Source: CAD feature listing. Evaluate the final solid. Frame: model axes, mm. A direction names the side the tool comes from. Round coordinates to 2 decimals unless told otherwise and drop trailing zeros. Loops run counter-clockwise (first coordinate to the right, second up) from the corner with the lowest first, then second, coordinate; pieces in that order, holes last. Notation, with made-up numbers: (28, 41) -> (39, 41) arc R22 ccw to (39, 50) -> close; hole circle Ø5 at (16.5, 22.5). An arc over 180 degrees is marked (long way). Put each result on its own line as item: value. Start each with the question number.
1. Set-up query: faces 1 (the flat face through (-115, -20.788, 3)), 2 (the flat face through (147.322, -24, 3)), 3 (the flat face through (100.927, -64, 3)). Return all of +Z, -Z, +X, -X, +Y, -Y with unobstructed straight access to the full face (end or side cutting, diameter ignored); none if empty.
2. Cut plane A-A (y = -42). Return the cut outline in (x, z), then the cut area to 3 significant figures.
3. Contact query for flat-ended pins moving along their axis: pin 1 (3 mm diameter, centred on y = -44, z = 3.5, fed in from +X); pin 2 (12 mm diameter, centred on x = -84, y = -61.5, fed in from -Z); pin 3 (1 mm diameter, centred on x = -8.5, z = 4.5, fed in from -Y); pin 4 (1.4 mm diameter, centred on y = -19, z = 1.5, fed in from -X). Output: stop coordinate, or through.
4. Draft query along X for faces 4 (the flat face through (-146.328, -53, 3)), 5 (the flat face through (153.672, -53, 3)), 6 (the cylindrical face through (89.507, -50.164, 3.219)). Return one class per face: pulls with the +X half, pulls with the -X half, needs draft (parallel to the pull), parting line crosses it, or undercut.
5. Cut plane B-B (x = 129). Return the cut outline in (y, z), then the cut area to 3 significant figures.
6. Material intervals for L1, parallel to X at y = -55, z = 0.75; L2, parallel to X at y = -64.5, z = 6.25; L3, parallel to X at y = -25, z = 2.25, sorted ascending.
```python
from build123d import *

# Parameters (mm, degrees)
BOSS_EXTRUDE1_DEPTH = 6.35
CUT_EXTRUDE2_DEPTH  = 169.008101823
CUT_EXTRUDE3_DEPTH  = 169.008101823
CUT_EXTRUDE4_DEPTH  = 169.008101823
FILLET1_R           = 0.254


with BuildPart() as part:
    # Model → Boss-Extrude1 (new body)
    with BuildSketch(Plane.XY):
        with BuildLine():
            Line((138.15521867, -67.612541882), (138.94896867, -66.818791882))
            Line((138.94896867, -66.818791882), (138.94896867, -62.385073899))
            ThreePointArc((138.94896867, -62.385073899), (138.948968669, -61.262541883), (140.071500684, -61.262541882))
            Line((140.071500684, -61.262541882), (140.971545702, -61.262541882))
            Line((140.971545702, -61.262541882), (140.971545702, -60.810273899))
            ThreePointArc((140.971545702, -60.810273899), (140.9715457, -59.687741883), (142.094077716, -59.687741882))
            Line((142.094077716, -59.687741882), (147.321545702, -59.687741882))
            Line((147.321545702, -59.687741882), (147.321545702, -58.735073899))
            ThreePointArc((147.321545702, -58.735073899), (147.3215457, -57.612541883), (148.444077716, -57.612541882))
            Line((148.444077716, -57.612541882), (152.084045702, -57.612541882))
            Line((152.084045702, -57.612541882), (153.671545702, -56.025041882))
            Line((153.671545702, -56.025041882), (153.671545702, -49.200041882))
            Line((153.671545702, -49.200041882), (152.084045702, -47.612541882))
            Line((152.084045702, -47.612541882), (148.444077716, -47.612541882))
            ThreePointArc((148.444077716, -47.612541882), (147.321545702, -47.612541882), (147.321545702, -46.490009867))
            Line((147.321545702, -46.490009867), (147.321545702, -38.735073899))
            ThreePointArc((147.321545702, -38.735073899), (147.3215457, -37.612541883), (148.444077716, -37.612541882))
            Line((148.444077716, -37.612541882), (152.084045702, -37.612541882))
            Line((152.084045702, -37.612541882), (153.671545702, -36.025041882))
            Line((153.671545702, -36.025041882), (153.671545702, -29.200041882))
            Line((153.671545702, -29.200041882), (152.084045702, -27.612541882))
            Line((152.084045702, -27.612541882), (148.444077716, -27.612541882))
            ThreePointArc((148.444077716, -27.612541882), (147.321545702, -27.612541882), (147.321545702, -26.490009867))
            Line((147.321545702, -26.490009867), (147.321545702, -20.787541882))
            Line((147.321545702, -20.787541882), (143.919077716, -20.787541882))
            ThreePointArc((143.919077716, -20.787541882), (142.796545702, -20.787541882), (142.796545702, -19.665009867))
            Line((142.796545702, -19.665009867), (142.796545702, -18.406291882))
            Line((142.796545702, -18.406291882), (142.002795702, -17.612541882))
            Line((142.002795702, -17.612541882), (133.590295702, -17.612541882))
            Line((133.590295702, -17.612541882), (132.796545702, -18.406291882))
            Line((132.796545702, -18.406291882), (132.796545702, -19.665009867))
            ThreePointArc((132.796545702, -19.665009867), (132.796545702, -20.787541882), (131.674013687, -20.787541882))
            Line((131.674013687, -20.787541882), (89.055077716, -20.787541882))
            ThreePointArc((89.055077716, -20.787541882), (87.932545702, -20.787541882), (87.932545702, -19.665009867))
            Line((87.932545702, -19.665009867), (87.932545702, -18.406291882))
            Line((87.932545702, -18.406291882), (87.138795702, -17.612541882))
            Line((87.138795702, -17.612541882), (78.726295702, -17.612541882))
            Line((78.726295702, -17.612541882), (77.932545702, -18.406291882))
            Line((77.932545702, -18.406291882), (77.932545702, -25.037209867))
            ThreePointArc((77.932545702, -25.037209867), (77.932545702, -26.159741882), (76.810013687, -26.159741882))
            Line((76.810013687, -26.159741882), (-69.46692228, -26.159741882))
            ThreePointArc((-69.46692228, -26.159741882), (-70.589454296, -26.159741883), (-70.589454297, -25.037209867))
            Line((-70.589454297, -25.037209867), (-70.589454297, -18.406291882))
            Line((-70.589454297, -18.406291882), (-71.383204297, -17.612541882))
            Line((-71.383204297, -17.612541882), (-79.795704297, -17.612541882))
            Line((-79.795704297, -17.612541882), (-80.589454297, -18.406291882))
            Line((-80.589454297, -18.406291882), (-80.589454297, -19.665009867))
            ThreePointArc((-80.589454297, -19.665009867), (-80.589454297, -20.787541882), (-81.711986312, -20.787541882))
            Line((-81.711986312, -20.787541882), (-100.521454296, -20.787541882))
            Line((-100.521454296, -20.787541882), (-100.521454296, -29.665009867))
            ThreePointArc((-100.521454296, -29.665009867), (-100.521454296, -30.787541882), (-101.64398631, -30.787541882))
            Line((-101.64398631, -30.787541882), (-104.398922281, -30.787541882))
            ThreePointArc((-104.398922281, -30.787541882), (-105.521454296, -30.787541882), (-105.521454296, -29.665009867))
            Line((-105.521454296, -29.665009867), (-105.521454296, -20.787541882))
            Line((-105.521454296, -20.787541882), (-124.33092228, -20.787541882))
            ThreePointArc((-124.33092228, -20.787541882), (-125.453454296, -20.787541883), (-125.453454297, -19.665009867))
            Line((-125.453454297, -19.665009867), (-125.453454297, -18.406291882))
            Line((-125.453454297, -18.406291882), (-126.247204297, -17.612541882))
            Line((-126.247204297, -17.612541882), (-134.659704297, -17.612541882))
            Line((-134.659704297, -17.612541882), (-135.453454297, -18.406291882))
            Line((-135.453454297, -18.406291882), (-135.453454297, -19.665009867))
            ThreePointArc((-135.453454297, -19.665009867), (-135.453454297, -20.787541882), (-136.575986312, -20.787541882))
            Line((-136.575986312, -20.787541882), (-139.978454297, -20.787541882))
            Line((-139.978454297, -20.787541882), (-139.978454297, -26.490009867))
            ThreePointArc((-139.978454297, -26.490009867), (-139.978454297, -27.612541882), (-141.100986312, -27.612541882))
            Line((-141.100986312, -27.612541882), (-144.740954297, -27.612541882))
            Line((-144.740954297, -27.612541882), (-146.328454297, -29.200041882))
            Line((-146.328454297, -29.200041882), (-146.328454297, -36.025041882))
            Line((-146.328454297, -36.025041882), (-144.740954297, -37.612541882))
            Line((-144.740954297, -37.612541882), (-141.100986312, -37.612541882))
            ThreePointArc((-141.100986312, -37.612541882), (-139.978454296, -37.612541883), (-139.978454297, -38.735073899))
            Line((-139.978454297, -38.735073899), (-139.978454297, -46.490009867))
            ThreePointArc((-139.978454297, -46.490009867), (-139.978454297, -47.612541882), (-141.100986312, -47.612541882))
            Line((-141.100986312, -47.612541882), (-144.740954297, -47.612541882))
            Line((-144.740954297, -47.612541882), (-146.328454297, -49.200041882))
            Line((-146.328454297, -49.200041882), (-146.328454297, -56.025041882))
            Line((-146.328454297, -56.025041882), (-144.740954297, -57.612541882))
            Line((-144.740954297, -57.612541882), (-141.100986312, -57.612541882))
            ThreePointArc((-141.100986312, -57.612541882), (-139.978454296, -57.612541883), (-139.978454297, -58.735073899))
            Line((-139.978454297, -58.735073899), (-139.978454297, -59.687741882))
            Line((-139.978454297, -59.687741882), (-134.750986312, -59.687741882))
            ThreePointArc((-134.750986312, -59.687741882), (-133.628454296, -59.687741883), (-133.628454297, -60.810273899))
            Line((-133.628454297, -60.810273899), (-133.628454297, -61.262541882))
            Line((-133.628454297, -61.262541882), (-132.630226339, -61.262541882))
            ThreePointArc((-132.630226339, -61.262541882), (-131.507694322, -61.262541882), (-131.507694322, -62.385073899))
            Line((-131.507694322, -62.385073899), (-131.507694322, -66.818791882))
            Line((-131.507694322, -66.818791882), (-130.713944322, -67.612541882))
            Line((-130.713944322, -67.612541882), (-128.072204297, -67.612541882))
            Line((-128.072204297, -67.612541882), (-127.278454297, -66.818791882))
            Line((-127.278454297, -66.818791882), (-127.278454297, -60.810273899))
            ThreePointArc((-127.278454297, -60.810273899), (-127.278454298, -59.687741883), (-126.155922283, -59.687741882))
            Line((-126.155922283, -59.687741882), (-94.70598631, -59.687741882))
            ThreePointArc((-94.70598631, -59.687741882), (-93.583454294, -59.687741883), (-93.583454296, -60.810273899))
            Line((-93.583454296, -60.810273899), (-93.583454296, -66.818791882))
            Line((-93.583454296, -66.818791882), (-92.789704296, -67.612541882))
            Line((-92.789704296, -67.612541882), (-89.377204296, -67.612541882))
            Line((-89.377204296, -67.612541882), (-88.583454296, -66.818791882))
            Line((-88.583454296, -66.818791882), (-88.583454296, -60.810273899))
            ThreePointArc((-88.583454296, -60.810273899), (-88.583454297, -59.687741883), (-87.460922281, -59.687741882))
            Line((-87.460922281, -59.687741882), (94.804013689, -59.687741882))
            ThreePointArc((94.804013689, -59.687741882), (95.926545704, -59.687741883), (95.926545703, -60.810273899))
            Line((95.926545703, -60.810273899), (95.926545703, -66.818791882))
            Line((95.926545703, -66.818791882), (96.720295703, -67.612541882))
            Line((96.720295703, -67.612541882), (100.132795703, -67.612541882))
            Line((100.132795703, -67.612541882), (100.926545703, -66.818791882))
            Line((100.926545703, -66.818791882), (100.926545703, -60.810273899))
            ThreePointArc((100.926545703, -60.810273899), (100.926545702, -59.687741883), (102.049077718, -59.687741882))
            Line((102.049077718, -59.687741882), (133.499013687, -59.687741882))
            ThreePointArc((133.499013687, -59.687741882), (134.621545703, -59.687741883), (134.621545702, -60.810273899))
            Line((134.621545702, -60.810273899), (134.621545702, -66.818791882))
            Line((134.621545702, -66.818791882), (135.415295702, -67.612541882))
            Line((135.415295702, -67.612541882), (138.15521867, -67.612541882))
        make_face()
    extrude(amount=BOSS_EXTRUDE1_DEPTH)

    # Sketch3 → Cut-Extrude2 (cut, through all)
    with BuildSketch(Plane.XY.offset(6.35)):
        with BuildLine():
            Line((-131.355294322, -62.171255574), (-131.355294322, -66.971191882))
            Line((-131.355294322, -66.971191882), (-131.507694322, -66.818791882))
            Line((-131.507694322, -66.818791882), (-131.507694322, -62.385073899))
            ThreePointArc((-131.507694322, -62.385073899), (-131.422591643, -62.284510162), (-131.355294322, -62.171255574))
        make_face()
        with BuildLine():
            Line((138.79656867, -62.171255574), (138.79656867, -66.971191882))
            Line((138.79656867, -66.971191882), (138.94896867, -66.818791882))
            Line((138.94896867, -66.818791882), (138.94896867, -62.385073899))
            ThreePointArc((138.94896867, -62.385073899), (138.86386599, -62.284510163), (138.79656867, -62.171255574))
        make_face()
    extrude(amount=-CUT_EXTRUDE2_DEPTH, mode=Mode.SUBTRACT)

    # Sketch4 → Cut-Extrude3 (cut, through all)
    with BuildSketch(Plane.XY.offset(6.35)):
        with BuildLine():
            Line((-85.408454296, -59.687741882), (-79.058454296, -59.687741882))
            Line((-79.058454296, -59.687741882), (-79.058454296, -53.337741882))
            ThreePointArc((-79.058454296, -53.337741882), (-82.233454296, -50.162741882), (-85.408454296, -53.337741882))
            Line((-85.408454296, -53.337741882), (-85.408454296, -59.687741882))
        make_face()
        with BuildLine():
            Line((86.4015457, -59.687741882), (86.4015457, -53.337741882))
            ThreePointArc((86.4015457, -53.337741882), (89.5765457, -50.162741882), (92.751545701, -53.337741882))
            Line((92.751545701, -53.337741882), (92.751545701, -59.687741882))
            Line((92.751545701, -59.687741882), (86.4015457, -59.687741882))
        make_face()
    extrude(amount=-CUT_EXTRUDE3_DEPTH, mode=Mode.SUBTRACT)

    # Sketch6 → Cut-Extrude4 (cut, through all)
    with BuildSketch(Plane.XY.offset(6.35)):
        with BuildLine():
            Line((-105.833547434, -30.787541882), (-105.833547434, -20.787541882))
            Line((-105.833547434, -20.787541882), (-100.209361158, -20.787541882))
            Line((-100.209361158, -20.787541882), (-100.209361158, -30.787541882))
            ThreePointArc((-100.209361158, -30.787541882), (-103.021454296, -33.59963502), (-105.833547434, -30.787541882))
        make_face()
    extrude(amount=-CUT_EXTRUDE4_DEPTH, mode=Mode.SUBTRACT)

    # Fillet1
    fillet1_edges = [part.edges().sort_by_distance(p)[0] for p in [
        (-85.408454296, -59.687741882, 3.175),
        (-79.058454296, -59.687741882, 3.175),
        (92.751545701, -59.687741882, 3.175),
        (86.4015457, -59.687741882, 3.175),
        (-105.833547434, -20.787541882, 3.175),
        (-100.209361158, -20.787541882, 3.175),
    ]]
    fillet(fillet1_edges, radius=FILLET1_R)


solid = part.part
```
Solution:
1. face 1: +Z, -Z, +Y
1. face 2: +Z, -Z, +X, +Y
1. face 3: +Z, -Z, -Y
2. outline: (-139.98, 0) -> (147.32, 0) -> (147.32, 6.35) -> (-139.98, 6.35) -> close
2. area: 1,820 mm^2
3. pin 1: stops at x = 147.32
3. pin 2: stops at z = 0
3. pin 3: stops at y = -59.69
3. pin 4: stops at x = -135.45
4. face 4: pulls with the -X half
4. face 5: pulls with the +X half
4. face 6: undercut
5. outline: (-59.69, 0) -> (-20.79, 0) -> (-20.79, 6.35) -> (-59.69, 6.35) -> close
5. area: 247 mm^2
6. L1: x = -146.33 to -85.41, -79.06 to 86.4, 92.75 to 153.67
6. L2: x = -131.36 to -127.28, -93.58 to -88.58, 95.93 to 100.93, 134.62 to 138.8
6. L3: x = -139.98 to -105.83, -100.21 to -70.59, 77.93 to 147.32
